Could you check a few things on this model? Use its own coordinates, in mm. Round coordinates to 2 decimals unless told otherwise and drop trailing zeros. Write each loop counter-clockwise with the first axis right and the second up, starting at its lowest first coordinate (ties: lowest second). Pieces come first, ordered by that corner, then holes. Notation, with made-up numbers: (-18.5, 79) -> (-10.5, 79) arc R27 cw to (-10.5, 115) -> close; hole circle Ø5 at (41.5, 45.5). An arc over 180 degrees is marked (long way). Return JSON: item names as keys, results as strings.
from build123d import *

# Parameters (mm, degrees)
EXTRUDE_1_DEPTH = 5
SKETCH_2_R      = 2.5
EXTRUDE_2_DEPTH = 50
EXTRUDE_3_DEPTH = 5


with BuildPart() as part:
    # 草图1 → 凸台-拉伸1 (new body)
    with BuildSketch(Plane.XY):
        with BuildLine():
            Line((-1, 3), (1, 3))
            Line((1, 3), (1, 2.291287847))
            ThreePointArc((1, 2.291287847), (0, -2.5), (-1, 2.291287847))
            Line((-1, 2.291287847), (-1, 3))
        make_face()
    extrude(amount=EXTRUDE_1_DEPTH)

    # 草图2 → 凸台-拉伸2 (add)
    with BuildSketch(Plane.XY.offset(5)):
        with Locations(Location((0, 0, 0), (0, 0, 113.578178478))):
            Circle(SKETCH_2_R)
    extrude(amount=EXTRUDE_2_DEPTH)

    # 草图3 → 凸台-拉伸3 (add)
    with BuildSketch(Plane.XY.offset(55)):
        with BuildLine():
            Line((-1, 3), (1, 3))
            Line((1, 3), (1, 2.291287847))
            ThreePointArc((1, 2.291287847), (0, -2.5), (-1, 2.291287847))
            Line((-1, 2.291287847), (-1, 3))
        make_face()
    extrude(amount=EXTRUDE_3_DEPTH)


solid = part.part
1) I want a section at B-B, the plane y = 1.65. Please give me the cut outline in (x, z), and give its area (3 significant figures).
Return value:
{"outline": "(-1.88, 0) -> (1.88, 0) -> (1.88, 60) -> (-1.88, 60) -> close", "area": "225 mm²"}
2) If I drill on probe 1 along Y at (x, z) = (-0.2, 30.5); probe 2 along Y at (x, z) = (0.8, 52), over which ranges is the centre line in solid material (lowest first)? Write a range as [from, to].
Return value:
{"probe 1": "[-2.49, 2.49]", "probe 2": "[-2.37, 2.37]"}
3) Will this pin go through, and if not, where does the flat tip stop? pin 1 Ø0.8 at (y, z) = (2.5, 2) entering from -X.
Return value:
{"pin 1": "x = -1.36"}
4) I want a section at C-C, the plane z = 29. Please give me the cut outline in (x, y).
Return value:
{"outline": "circle Ø5 at (0, 0)"}
5) I want a section at A-A, the plane x = 0. Please give me the cut outline in (y, z).
Return value:
{"outline": "(-2.5, 0) -> (3, 0) -> (3, 5) -> (2.5, 5) -> (2.5, 55) -> (3, 55) -> (3, 60) -> (-2.5, 60) -> close"}
